Build history of the part. All positions in model axes, mm. A direction names the side the tool comes from. Coordinates: 2 decimals unless noted, no trailing zeros. Write each loop counter-clockwise with the first axis right and the second up, starting at its lowest first coordinate (ties: lowest second). Pieces come first, ordered by that corner, then holes.
from build123d import *

# Parameters (mm, degrees)
PAD_DEPTH = 1


with BuildPart() as part:
    # Sketch → Pad (new body)
    with BuildSketch(Plane.XY):
        with BuildLine():
            Line((3, 0), (-3, 0))
            Line((-3, 0), (-2.687677, 3.257669))
            ThreePointArc((-2.687677, 3.257669), (-2.954386, 4.423147), (-3.838312, 5.228222))
            ThreePointArc((-1.148945, 9.886566), (-5.038297, 9.026488), (-3.838312, 5.228222))
            ThreePointArc((-1.148945, 9.886566), (-6e-06, 9.523614), (1.148936, 9.88656))
            ThreePointArc((3.838472, 5.228297), (5.03825, 9.02657), (1.148936, 9.88656))
            ThreePointArc((3.838472, 5.228297), (2.946118, 4.408497), (2.690913, 3.223914))
            Line((3, 0), (2.690913, 3.223914))
        make_face()
    extrude(amount=PAD_DEPTH)


solid = part.part
(1) 3-axis set-ups, long thin cutter, end or side, ignore diameter. For faces 1 (the flat face through (2.848, 1.589, 0.493)), 2 (the flat face through (0, 5, 1)), 3 (the flat face through (-2.846, 1.606, 0.493)): which of +Z, -Z, +X, -X, +Y, -Y reach the whole face in a straight line?
(2) Slice it at A-A, the plane z = 0.6. List the corners of the cut face in (x, y), and give its area (3 significant figures).
(3) Slice it at B-B, the plane x = 0. List the corners of the cut face in (y, z).
(4) Slice it at C-C, the plane y = 3.5. List the corners of the cut face in (x, z).
(5) Two-plate mould, pull along X, no slides. Class faces 4 (the cylindrical face through (2.955, 4.423, 0.493)), 5 (the flat face through (0, 5, 0)), 6 (the cylindrical face through (5.07, 8.97, 0.49)): pulls with the +X half, pulls with the -X half, needs draft (parallel to the pull), parting line crosses it, or undercut.
(6) Probe L1, parallel to Y at x = 0, z = 0.55; L2, parallel to X at y = 4.5, z = 0.3; L3, parallel to X at y = 7.75, z = 0.95. List the from-to ranges inside material, lowest first.
Results:
1. face 1: +Z, -Z, +X
1. face 2: +Z, +X, -X, +Y, -Y
1. face 3: +Z, -Z, -X
2. outline: (-3.84, 5.23) arc R2 cw to (-2.69, 3.26) - (-3, 0) - (3, 0) - (2.69, 3.22) arc R2 cw to (3.84, 5.23) arc R2.7 ccw (long way) to (1.15, 9.89) arc R2 cw to (-1.15, 9.89) arc R2.7 ccw (long way) to start
2. area: 78.4 mm2
3. outline: (0, 0) - (9.52, 0) - (9.52, 1) - (0, 1) - close
4. outline: (-2.68, 0) - (2.68, 0) - (2.68, 1) - (-2.68, 1) - close
5. face 4: pulls with the +X half
5. face 5: needs draft
5. face 6: undercut
6. L1: y = 0 to 9.52
6. L2: x = -3 to 3
6. L3: x = -5.4 to 5.4
